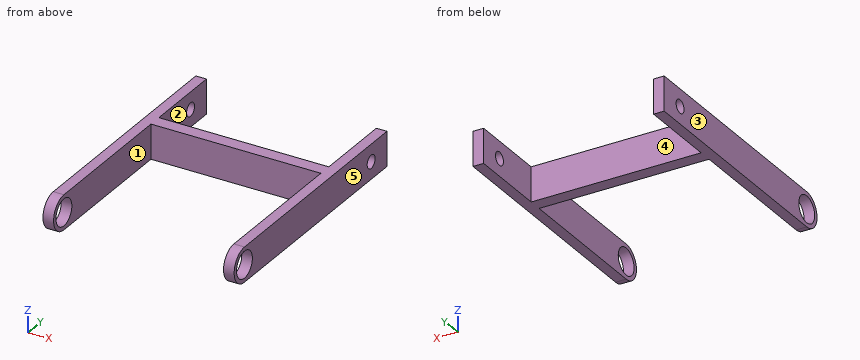
from build123d import *

# Parameters (mm, degrees)
BOSS_EXTRU_1_DEPTH      = 13
ESQUISSE2_R             = 5
ENL_V_MAT_EXTRU_1_DEPTH = 124.907223357
ESQUISSE3_R             = 2.5
ENL_V_MAT_EXTRU_2_DEPTH = 124.907223357
ENL_V_MAT_EXTRU_4_DEPTH = 124.907223357


with BuildPart() as part:
    # Esquisse1 → Boss.-Extru.1 (new body)
    with BuildSketch(Plane.XY):
        Polygon((0, 0), (0, 100), (4, 100), (4, 70), (68, 70), (68, 100), (72, 100), (72, 0), (68, 0), (68, 65), (4, 65), (4, 0), align=None)
    extrude(amount=BOSS_EXTRU_1_DEPTH)

    # Esquisse2 → Enlèv. mat.-Extru.1 (cut, through all)
    with BuildSketch(Plane(origin=(72, 0, 0), x_dir=(0, 0, -1), z_dir=(1, 0, 0))):
        with Locations(Location((-6.5, 10.1, 0), (0, 0, 90))):
            Circle(ESQUISSE2_R)
    extrude(amount=-ENL_V_MAT_EXTRU_1_DEPTH, mode=Mode.SUBTRACT)

    # Esquisse3 → Enlèv. mat.-Extru.2 (cut, through all)
    with BuildSketch(Plane.ZY):
        with Locations((6.5, 90)):
            Circle(ESQUISSE3_R)
    extrude(amount=-ENL_V_MAT_EXTRU_2_DEPTH, mode=Mode.SUBTRACT)

    # Esquisse5 → Enlèv. mat.-Extru.4 (cut, through all)
    with BuildSketch(Plane.ZY):
        with BuildLine():
            Line((0, 10.1), (0, -2.98091379))
            Line((0, -2.98091379), (15.001453012, -2.98091379))
            Line((15.001453012, -2.98091379), (15.001453012, 10.1))
            Line((15.001453012, 10.1), (13, 10.1))
            ThreePointArc((13, 10.1), (6.5, 3.6), (0, 10.1))
        make_face()
    extrude(amount=-ENL_V_MAT_EXTRU_4_DEPTH, mode=Mode.SUBTRACT)


solid = part.part
For this review, take the finished solid that the model builds, in its own axes (mm). Face numbers are marked on the shaded views. A direction names the side the tool comes from. Give positions to 0.01 mm unless a question says otherwise; leave off trailing zeros. Loops run counter-clockwise (first coordinate to the right, second up) from the corner with the lowest first, then second, coordinate; pieces in that order, holes last. Notation, with made-up numbers: (2.5, 23.5) -> (43.5, 23.5) arc R23 ccw to (43.5, 43.5) -> close; hole circle Ø11 at (46, -1.5). An arc over 180 degrees is marked (long way). One line per question, with ' | ' between items.
1) We need section B-B (z = 6.5). Write out the cut boundary in (x, y).
Resolved:
outline: (0, 3.6) -> (4, 3.6) -> (4, 5.1) -> (0, 5.1) -> close; (0, 15.1) -> (4, 15.1) -> (4, 65) -> (68, 65) -> (68, 15.1) -> (72, 15.1) -> (72, 87.5) -> (68, 87.5) -> (68, 70) -> (4, 70) -> (4, 87.5) -> (0, 87.5) -> close; (0, 92.5) -> (4, 92.5) -> (4, 100) -> (0, 100) -> close; (68, 3.6) -> (72, 3.6) -> (72, 5.1) -> (68, 5.1) -> close; (68, 92.5) -> (72, 92.5) -> (72, 100) -> (68, 100) -> close
2) For the marked faces 1 and 2, list the 3-axis set-ups (+Z, -Z, +X, -X, +Y, -Y) from which the entire face can be reached by the end or side of a thin tool; tool diameter is ignored.
Resolved:
face 1: +Z, -Z, -Y | face 2: +Z, -Z, +Y
3) To check wall thickness, follow probe 1 along X at (y, z) = (86.5, 10.5); probe 2 along Z at (x, y) = (2.6, 10.1); probe 3 along Y at (x, z) = (36.5, 12.25). State the ranges of each line that lie inside material, in increasing order.
Resolved:
probe 1: x = 0 to 4, 68 to 72 | probe 2: z = 0 to 1.5, 11.5 to 13 | probe 3: y = 65 to 70
4) We need section C-C (y = 90). Write out the cut boundary in (x, z).
Resolved:
outline: (0, 0) -> (4, 0) -> (4, 4) -> (0, 4) -> close; (0, 9) -> (4, 9) -> (4, 13) -> (0, 13) -> close; (68, 0) -> (72, 0) -> (72, 4) -> (68, 4) -> close; (68, 9) -> (72, 9) -> (72, 13) -> (68, 13) -> close
5) Insertion check: pin 1 Ø5 at (y, z) = (52.5, 5.5) entering from -X; pin 2 Ø4 at (x, z) = (11.5, 6) entering from -Y. Each pin has a flat end and moves straight along its axis. Give the tip position at first contact, or say it passes through.
Resolved:
pin 1: stops at x = 0 | pin 2: stops at y = 65
6) We need section A-A (y = 27). Write out the cut boundary in (x, z).
Resolved:
outline: (0, 0) -> (4, 0) -> (4, 13) -> (0, 13) -> close; (68, 0) -> (72, 0) -> (72, 13) -> (68, 13) -> close
7) The part is to be moulded in two halves that separate along X. For the marked faces 3, 4 and 5, say which applies: +X half, -X half, draft (parallel to the pull), parting line (faces both ways), or undercut.
Resolved:
face 3: -X half | face 4: undercut | face 5: +X half
8) We need section D-D (x = 47). Write out the cut boundary in (y, z), plus the area to 3 significant figures.
Resolved:
outline: (65, 0) -> (70, 0) -> (70, 13) -> (65, 13) -> close | area: 65.0 mm2
